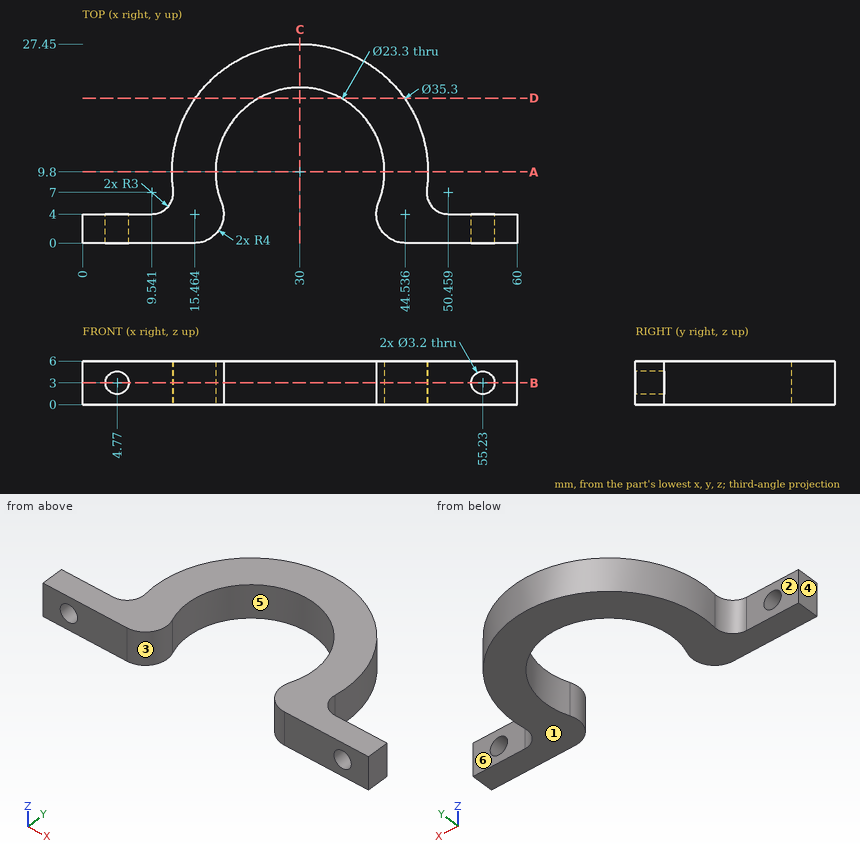
Here's the drawing with two shaded views (mm, measured from the low corner). I have some questions. A direction names the side the tool comes from. Coordinates: 2 decimals unless noted, no trailing zeros. Order: outer loops, then holes, each group sorted by start corner. A loop starts at its lowest first (then second) coordinate and runs counter-clockwise, first axis right, second up.
Item 1: For the marked faces 1, 2 and 3, which set-ups out of +Z, -Z, +X, -X, +Y, -Y let a thin tool reach every point of the face, with its end or its side?
Result sheet:
face 1: -Z, +X, -X, +Y, -Y
face 2: +Z, -Z, -X, +Y
face 3: +Z, -Z
Item 2: For P1, Ø12, axis at x = 28, y = 12.5, coming from the +Z side; P2, Ø1.8, axis at x = 6, z = 4.5, coming from the +Y side; P3, Ø3, axis at y = 9.5, z = 3.5, coming from the +X side; P4, Ø1, axis at x = 49, z = 4, coming from the +Y side, each with a flat end and sliding along its axis, tell me the tip position at first contact or that it passes through.
Result sheet:
P1: passes through
P2: stops at y = 4
P3: stops at x = 47.65
P4: stops at y = 4.73
Item 3: I need wall thicknesses on line 1 (X direction, y = 0.9, z = 3) (1 decimal); line 2 (X direction, y = 9.8, z = 3.6); line 3 (X direction, y = 5, z = 1.8) (1 decimal). Which ranges of each line are inside material? Lowest first, please.
Result sheet:
line 1: x = 0 to 3.2, 6.4 to 18, 42 to 53.6, 56.8 to 60
line 2: x = 12.35 to 18.35, 41.65 to 47.65
line 3: x = 11.8 to 19.3, 40.7 to 48.2
Item 4: If we section it at A-A on y = 9.8: List the corners of the cut face in (x, z) for me, plus the area to 3 significant figures.
Result sheet:
outline: (12.35, 0) - (18.35, 0) - (18.35, 6) - (12.35, 6) - close; (41.65, 0) - (47.65, 0) - (47.65, 6) - (41.65, 6) - close
area: 72.0 mm2
Item 5: If we section it at C-C on x = 30: List the corners of the cut face in (y, z) for me, plus the area to 3 significant figures.
Result sheet:
outline: (21.45, 0) - (27.45, 0) - (27.45, 6) - (21.45, 6) - close
area: 36.0 mm2
Item 6: If we section it at B-B on z = 3: State how many separate pieces and enclosed holes the cut face has, plus the area to 3 significant figures.
Result sheet:
separate pieces: 3
enclosed holes: 0
area: 477 mm2
Item 7: If we section it at D-D on y = 20: List the corners of the cut face in (x, z) for me (1 decimal).
Result sheet:
outline: (15.6, 0) - (24.4, 0) - (24.4, 6) - (15.6, 6) - close; (35.6, 0) - (44.4, 0) - (44.4, 6) - (35.6, 6) - close
Item 8: If we mould it in two halves opening along Y, with no side actions, what happens to the marked faces 4, 5 and 6? For each: +Y half, -Y half, draft (parallel to the pull), parting line (faces both ways), or undercut.
Result sheet:
face 4: draft
face 5: undercut
face 6: +Y half
